Can you work these out from the model? Positions are in its coordinate system, mm. A direction names the side the tool comes from. Round coordinates to 2 decimals unless told otherwise and drop trailing zeros. Order: outer loops, then holes, each group sorted by start corner. A loop starts at its lowest first (then second) coordinate and runs counter-clockwise, first axis right, second up.
from build123d import *

# Parameters (mm, degrees)
BOSS_EXTRUDE1_DEPTH = 27
SKETCH4_R           = 1.5
CUT_EXTRUDE1_DEPTH  = 10


with BuildPart() as part:
    # Sketch1 → Revolve1 (revolve)
    with BuildSketch(Plane(origin=(0, 0, 0), x_dir=(0, 0, -1), z_dir=(1, 0, 0)), mode=Mode.PRIVATE) as revolve1_sk:
        Polygon((0, 0), (0, 19), (75, 19), (75, 6.25), (76.5, 6.25), (76.5, 2.5), (101.5, 2.5), (101.5, 0), align=None)
    revolve(revolve1_sk.sketch.rotate(Axis((0, 0, 0), (0, 0, -1)), 90), axis=Axis((0, 0, 0), (0, 0, -1)))

    # Sketch2 → Boss-Extrude1 (add)
    with BuildSketch(Plane.XY):
        with BuildLine():
            Line((-19, 0), (-19, 25.5))
            ThreePointArc((-19, 25.5), (-18.267766953, 27.267766953), (-16.5, 28))
            Line((-16.5, 28), (16.5, 28))
            ThreePointArc((16.5, 28), (18.267766953, 27.267766953), (19, 25.5))
            Line((19, 25.5), (19, 0))
            ThreePointArc((19, 0), (0, -19), (-19, 0))
        make_face()
    extrude(amount=BOSS_EXTRUDE1_DEPTH)

    # Sketch4 → Cut-Extrude1 (cut)
    with BuildSketch(Plane(origin=(0, 0, -75), x_dir=(-1, 0, 0), z_dir=(0, 0, -1))):
        with Locations((-8.838834765, 8.838834765)):
            Circle(SKETCH4_R)
        with Locations((8.838834765, 8.838834765)):
            Circle(SKETCH4_R)
        with Locations((8.838834765, -8.838834765)):
            Circle(SKETCH4_R)
        with Locations((-8.838834765, -8.838834765)):
            Circle(SKETCH4_R)
    extrude(amount=-CUT_EXTRUDE1_DEPTH, mode=Mode.SUBTRACT)


solid = part.part
(1) On a 3-axis mill with a long thin cutter (end or side, diameter ignored), from which of +Z, -Z, +X, -X, +Y, -Y can I reach the whole of each face in a straight line? I mean faces 4 (the face through (0, 20, 0)), 5 (the face through (5.96, -1.88, -75.76)), 6 (the face through (18.248, 27.287, 13.311)). Say none if no direction works.
(2) If we mould it in two halves opening along X, with no side actions, what happens to faces 1 (the face through (10.03, 7.93, -70.07)), 2 (the face through (-2.5, -0.1, -89.2)), 3 (the face through (8, 0, -75))? For each: pulls with the +X half, pulls with the -X half, needs draft (parallel to the pull), parting line crosses it, or undercut.
(3) I want a section at B-B, the plane z = 4. List the corners of the cut face in (x, y) for me.
(4) Please list where these lines run through material, in increasing order: probe 1 along Z at (x, y) = (7, 25); probe 2 along Z at (x, y) = (-4, -3.5); probe 3 along Y at (x, z) = (0.5, 18.5).
(5) I want a section at A-A, the plane x = 0. List the corners of the cut face in (y, z) for me.
(6) I want a section at D-D, the plane y = 14. List the corners of the cut face in (x, z) for me, plus the area to 3 significant figures.
(7) I want a section at C-C, the plane z = -69.5. List the corners of the cut face in (x, y) for me.
(8) I'm going to push flat-ended pins straight in: pin 1 Ø2.5 at (x, y) = (8.5, -9) entering from -Z; pin 2 Ø1.5 at (x, y) = (-8.5, 9) entering from -Z; pin 3 Ø4 at (x, y) = (-14.5, 17) entering from -Z; pin 4 Ø1 at (x, z) = (7.5, -77.5) entering from -Y. Where does each tip first touch, or does it pass through?
Ans:
1. face 4: -Z, +Y
1. face 5: -Z
1. face 6: +Z, -Z, +X, +Y
2. face 1: undercut
2. face 2: parting line crosses it
2. face 3: needs draft
3. outline: (-19, 0) arc R19 ccw to (19, 0) - (19, 25.5) arc R2.5 ccw to (16.5, 28) - (-16.5, 28) arc R2.5 ccw to (-19, 25.5) - close
4. probe 1: z = 0 to 27
4. probe 2: z = -76.5 to 27
4. probe 3: y = -18.99 to 28
5. outline: (-19, -75) - (-6.25, -75) - (-6.25, -76.5) - (-2.5, -76.5) - (-2.5, -101.5) - (2.5, -101.5) - (2.5, -76.5) - (6.25, -76.5) - (6.25, -75) - (19, -75) - (19, 0) - (28, 0) - (28, 27) - (-19, 27) - close
6. outline: (-19, 0) - (-12.85, 0) - (-12.85, -75) - (12.85, -75) - (12.85, 0) - (19, 0) - (19, 27) - (-19, 27) - close
6. area: 2,950 mm2
7. outline: circle Ø38 at (0, 0); hole circle Ø3 at (-8.84, -8.84); hole circle Ø3 at (-8.84, 8.84); hole circle Ø3 at (8.84, -8.84); hole circle Ø3 at (8.84, 8.84)
8. pin 1: stops at z = -75
8. pin 2: stops at z = -65
8. pin 3: stops at z = 0
8. pin 4: passes through
